Autodesk Fusion 360 part; units mm, degrees
sketch "Sketch1" plane through (0, 0, 0) normal (0, 1, 0) x (1, 0, 0)
  line L0 (0, 0) -> (0, -240)
  line L1 (0, 0) -> (30, 0)
  line L2 (30, 0) -> (30, -130)
  spline S0 degree 5 poles (30, -130) (29.9765, -130.5738) (29.9204, -131.6926) (29.8084, -133.2846) (29.6036, -135.235) (29.2504, -137.391) (28.7863, -139.284) (28.1857, -140.9528) (27.4028, -142.4662) (26.3864, -143.9173) (25.1131, -145.4043) (23.6149, -147.0156) (22.0109, -148.8121) (20.4671, -150.8302) (19.151, -153.0839) (18.1911, -155.5676) (17.6291, -158.2582) (17.3904, -161.1182) (17.3386, -164.106) (17.3136, -167.1843) (17.1813, -170.3303) (16.8672, -173.5425) (16.4268, -176.856) (15.8829, -180.3105) (15.2457, -183.9433) (14.5178, -187.7806) (13.7043, -191.8294) (12.8205, -196.0692) (11.9002, -200.4438) (11.0056, -204.8517) (10.2328, -209.1403) (9.6869, -213.1347) (9.4586, -216.6645) (9.6016, -219.5898) (10.1061, -221.8312) (10.8818, -223.3904) (11.5446, -224.1973) (12.0407, -224.5695) (12.3702, -224.7147) (12.5347, -224.7615) knots 0 0 0 0 0 0 0.028571 0.057143 0.085714 0.114286 0.142857 0.171429 0.2 0.228571 0.257143 0.285714 0.314286 0.342857 0.371429 0.4 0.428571 0.457143 0.485714 0.514286 0.542857 0.571429 0.6 0.628571 0.657143 0.685714 0.714286 0.742857 0.771429 0.8 0.828571 0.857143 0.885714 0.914286 0.942857 0.971429 1 1 1 1 1 1
  spline S1 degree 5 poles (12.5347, -224.7615) (12.5672, -225.1026) (12.605, -225.796) (12.5803, -226.8697) (12.387, -228.3526) (11.9068, -230.1993) (11.2582, -231.9222) (10.5553, -233.4058) (10.003, -234.5642) (9.843, -235.3668) (10.5718, -235.8733) (11.6234, -236.2748) (12.1639, -236.7697) (11.9167, -237.4572) (11.6619, -238.2348) (11.2194, -239.0006) (10.4447, -239.5113) (9.4203, -239.7979) (8.5112, -239.9407) (8, -240) knots 0 0 0 0 0 0 0.066667 0.133333 0.2 0.266667 0.333333 0.4 0.466667 0.533333 0.6 0.666667 0.733333 0.8 0.866667 0.933333 1 1 1 1 1 1
  line L3 (17.898, -162.5327) -> (16.102, -181.4673)
  line L4 (7.9977, -216.9977) -> (12.9977, -227.9977)
  line L5 (12.3644, -222.9737) -> (12.7049, -226.5494)
  line L6 (10, -234) -> (10, -236)
  line L7 (12, -236) -> (12, -238)
  line L8 (11.8794, -239.5497) -> (4.1206, -240.4503)
  line L9 (8, -240) -> (0, -240)
  point P0 (28.5, -140)
  point P1 (25, -145.5)
  point P2 (18.454, -155.0935)
  point P3 (17, -172)
  point P4 (12, -200)
  point P5 (10.4977, -222.4977)
  point P6 (10, -235)
  point P7 (12, -237)
  dimension "d1" = 240
  dimension "d2" = 30
  dimension "d3" = 90
  dimension "d4" = 130
sketch "Sketch2" plane through (0, 0, 0) normal (0, 1, 0) x (1, 0, 0)
revolve "Revolve1" add sketch "Sketch1" angle 360 about axis through (0, 0, 0) along (0, 0, 1)
fillet "Fillet1" radius 1.5 1 edges at (-11.6864, -4.5327, 224.7615)
shell "Shell1" thickness 0.75 removed faces 1 at (-2.2732, -5.7921, 240)
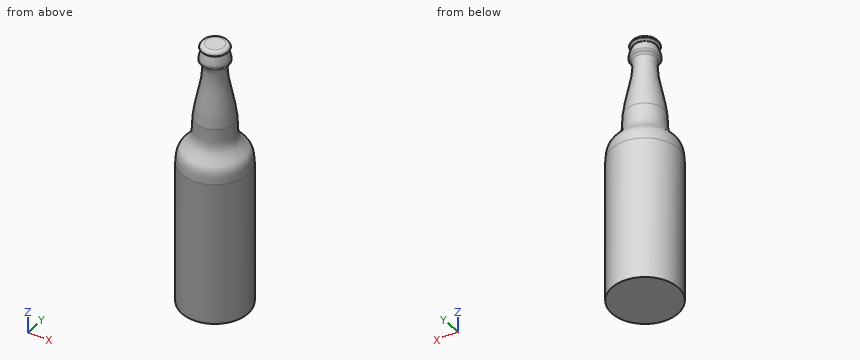
Input: part model. Units: mm. Frame: model coordinates. Give positions to 0.01 mm unless a question says otherwise; leave off trailing zeros. Write each loop counter-clockwise with the first axis right and the second up, starting at its lowest first coordinate (ties: lowest second). Pieces come first, ordered by that corner, then holes.
Q1. Section A-A, the plane z = 21.5. Output: boundary loops of the cut face in (x, y).
Q2. First-contact query: P1, Ø6, axis at y = -22, z = 50.5, coming from the +X side; P2, Ø4, axis at y = 3.5, z = 117.5, coming from the -X side; P3, Ø2, axis at y = -3.5, z = 212, coming from the -X side; P4, Ø5, axis at x = -16, y = 6, coming from the -Z side. Flat tips, straight axial feed; report the tip coordinate or a pass-through.
Q3. Material intervals for probe 1 along X at (y, z) = (-1.5, 107.5); probe 2 along X at (y, z) = (-25.5, 51); probe 3 along Y at (x, z) = (9, 37), sorted ascending.
Filled in:
1. outline: circle Ø60 at (0, 0)
2. P1: stops at x = 23.22
2. P2: stops at x = -29.96
2. P3: stops at x = -9.59
2. P4: stops at z = 0
3. probe 1: x = -29.96 to 29.96
3. probe 2: x = -15.8 to 15.8
3. probe 3: y = -28.62 to 28.62
